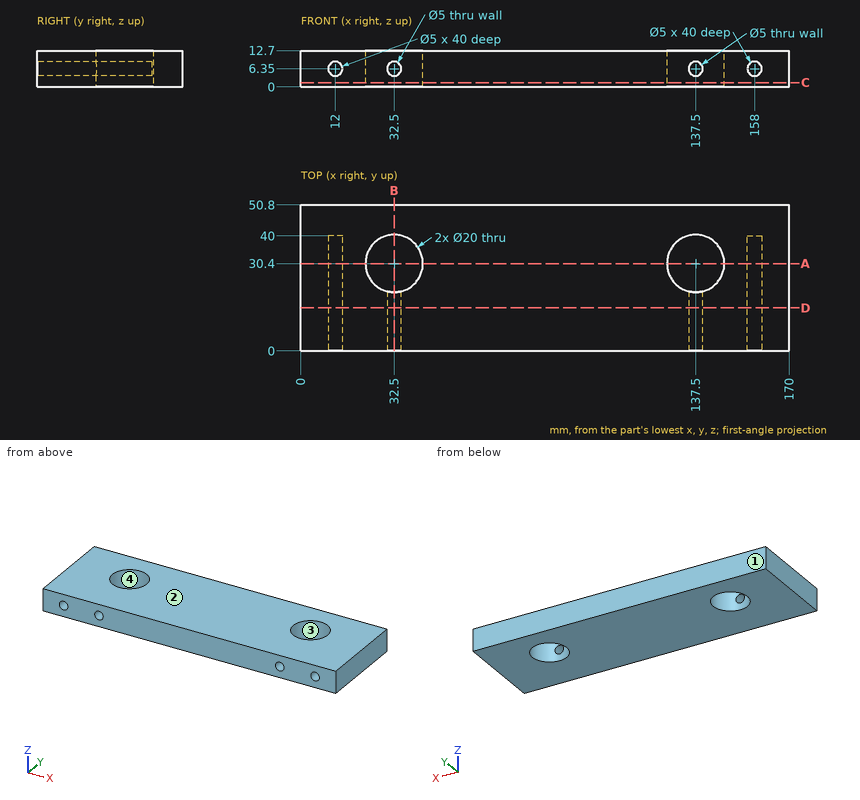
Check sheet for the drawn part. Datum: minimum x, y, z corner. Units: mm. Round coordinates to 2 decimals unless told otherwise and drop trailing zeros. Write each loop counter-clockwise with the first axis right and the second up, starting at its lowest first coordinate (ties: lowest second). Pieces come first, ordered by that corner, then holes. Notation, with made-up numbers: (41.5, -3) -> (68.5, -3) arc R33 ccw to (68.5, 31) -> close; hole circle Ø1 at (43.5, 68.25). An arc over 180 degrees is marked (long way). Write each question's results on one line, items separated by ' | '. Start each with the question number.
1. Draft check along Y on the marked faces 1, 2, 3 and 4. Enter one of: +Y half, -Y half, draft (parallel to the pull), parting line (faces both ways), or undercut.
2. Material ranges on probe 1 along Z at (x, y) = (12, 20.5); probe 2 along X at (y, z) = (4, 8.5); probe 3 along X at (y, z) = (29.5, 1.75), recorded low to high. Write a range as from..to.
3. Cross-section at C-C (z = 1.5). Enter the section's corners in (x, y).
4. Cross-section at D-D (y = 15). Enter the section's corners in (x, z).
5. Cross-section at B-B (x = 32.5). Enter the section's corners in (y, z).
6. Depth check by flat-ended pin: P1, Ø4.5, axis at x = 158, z = 6.35, coming from the -Y side; P2, Ø3, axis at x = 137.5, z = 6.35, coming from the -Y side. Enter the tip coordinate at first touch or a pass-through.
7. Cross-section at A-A (y = 30.4). Enter the section's corners in (x, z), then the cut area to 3 significant figures.
Solutions:
1) face 1: +Y half | face 2: draft | face 3: undercut | face 4: undercut
2) probe 1: z = 0..3.85, 8.85..12.7 | probe 2: x = 0..10.72, 13.28..31.22, 33.78..136.22, 138.78..156.72, 159.28..170 | probe 3: x = 0..22.54, 42.46..127.54, 147.46..170
3) outline: (0, 0) -> (170, 0) -> (170, 50.8) -> (0, 50.8) -> close; hole circle Ø20 at (32.5, 30.4); hole circle Ø20 at (137.5, 30.4)
4) outline: (0, 0) -> (170, 0) -> (170, 12.7) -> (0, 12.7) -> close; hole circle Ø5 at (12, 6.35); hole circle Ø5 at (32.5, 6.35); hole circle Ø5 at (137.5, 6.35); hole circle Ø5 at (158, 6.35)
5) outline: (0, 0) -> (20.4, 0) -> (20.4, 3.85) -> (0, 3.85) -> close; (0, 8.85) -> (20.4, 8.85) -> (20.4, 12.7) -> (0, 12.7) -> close; (40.4, 0) -> (50.8, 0) -> (50.8, 12.7) -> (40.4, 12.7) -> close
6) P1: stops at y = 40 | P2: stops at y = 40.29
7) outline: (0, 0) -> (22.5, 0) -> (22.5, 12.7) -> (0, 12.7) -> close; (42.5, 0) -> (127.5, 0) -> (127.5, 12.7) -> (42.5, 12.7) -> close; (147.5, 0) -> (170, 0) -> (170, 12.7) -> (147.5, 12.7) -> close; hole circle Ø5 at (12, 6.35); hole circle Ø5 at (158, 6.35) | area: 1,610 mm2
